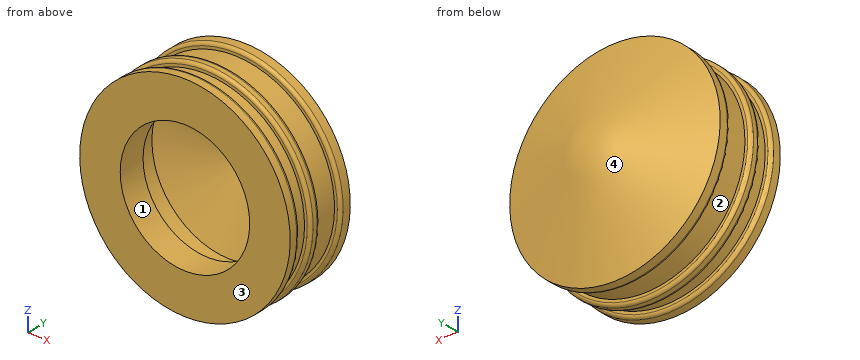
from build123d import *

# Parameters (mm, degrees)
SKETCH3_R          = 13.25
SKETCH3_R_2        = 12.5
CUT_EXTRUDE1_DEPTH = 1.7
SKETCH4_R          = 13.25
SKETCH4_R_2        = 12.5
CUT_EXTRUDE2_DEPTH = 3.2
FILLET1_R          = 0.4


with BuildPart() as part:
    # Sketch2 → Revolve1 (revolve)
    with BuildSketch(Plane(origin=(0, 0, 0), x_dir=(0, 0, -1), z_dir=(1, 0, 0))):
        Polygon((0, 14.3), (13.25, 9.2), (13.25, 0), (8.15, 0), (8.15, 3.5), (9.75, 3.5), (9.75, 6.796854291), (0, 10.54968448), align=None)
    revolve(axis=Axis((0, -0.715, 0), (0, 1, 0)))

    # Sketch3 → Cut-Extrude1 (cut)
    with BuildSketch(Plane(origin=(0, 1.4, 0), x_dir=(1, 0, 0), z_dir=(0, 1, 0))):
        with Locations(Location((0, 0, 0), (0, 0, 90))):
            Circle(SKETCH3_R)
        with Locations(Location((0, 0, 0), (0, 0, 270))):
            Circle(SKETCH3_R_2, mode=Mode.SUBTRACT)
    extrude(amount=CUT_EXTRUDE1_DEPTH, mode=Mode.SUBTRACT)

    # Sketch4 → Cut-Extrude2 (cut)
    with BuildSketch(Plane(origin=(0, 4.5, 0), x_dir=(1, 0, 0), z_dir=(0, 1, 0))):
        with Locations(Location((0, 0, 0), (0, 0, 270))):
            Circle(SKETCH4_R)
        with Locations(Location((0, 0, 0), (0, 0, 270))):
            Circle(SKETCH4_R_2, mode=Mode.SUBTRACT)
    extrude(amount=CUT_EXTRUDE2_DEPTH, mode=Mode.SUBTRACT)

    # Fillet1
    fillet1_edges = [part.edges().sort_by_distance(p)[0] for p in [
        (0, 3.1, 13.25),
        (0, 1.4, 13.25),
        (0, 7.7, 13.25),
        (0, 4.5, 13.25),
    ]]
    fillet(fillet1_edges, radius=FILLET1_R)


solid = part.part
For this review, take the finished solid that the model builds, in its own axes (mm). Face numbers are marked on the shaded views. Round coordinates to 2 decimals unless told otherwise and drop trailing zeros. Write each loop counter-clockwise with the first axis right and the second up, starting at its lowest first coordinate (ties: lowest second). Pieces come first, ordered by that corner, then holes. Notation, with made-up numbers: (46, -21) - (64, -21) arc R20 cw to (64, 6) - close; hole circle Ø6 at (3, 61.25). An arc over 180 degrees is marked (long way). Write item = value, one per line. Start each with the question number.
1. Wall thickness on L1, parallel to X at y = 4.7, z = 0; L2, parallel to Z at x = 0, y = 4.3; L3, parallel to X at y = 4.25, z = 4.25: over which ranges is each line inside the solid? List them lowest first.
2. Draft analysis for pull direction Y (two halves, no side actions). For the marked faces 1, 2, 3 and 4, state which applies: released by +Y, released by -Y, zero draft, split by the parting line, or undercut.
3. For pin 1 Ø8 at (x, z) = (-2, -10.5) entering from +Y; pin 2 Ø1.5 at (x, y) = (10, 5) entering from +Z; pin 3 Ø2 at (y, z) = (9.5, 8) entering from -X, all flat-tipped, find the tip position at first contact; note any pin that passes through.
4. Consider section A-A on y = 2. State the section outline as (x, z) points.
Evaluation:
q1.L1 = -12.5 to -9.75, 9.75 to 12.5
q1.L2 = -13.2 to -9.75, 9.75 to 13.2
q1.L3 = -12.52 to -8.77, 8.77 to 12.52
q2.face_1 = zero draft
q2.face_2 = undercut
q2.face_3 = released by -Y
q2.face_4 = released by +Y
q3.pin_1 = 11.73
q3.pin_2 = 8.99
q3.pin_3 = -11.22
q4.outline = circle Ø25 at (0, 0); hole circle Ø16.3 at (0, 0)
